from build123d import *

# Parameters (mm, degrees)
SKETCH_1_W     = 40
SKETCH_1_H     = 1.4
CHAMFER_1_SIZE = 0.2


with BuildPart() as part:
    # ｽｹｯﾁ1 → 回転1 (revolve)
    with BuildSketch(Plane(origin=(0, 0, 0), x_dir=(0, 0, -1), z_dir=(1, 0, 0)), mode=Mode.PRIVATE) as revolve_1_sk:
        with Locations((0, 2.3)):
            Rectangle(SKETCH_1_W, SKETCH_1_H)
    revolve(revolve_1_sk.sketch.rotate(Axis((0, 0, 7.128099174), (0, 0, -1)), 90), axis=Axis((0, 0, 7.128099174), (0, 0, -1)))

    # 面取り1
    chamfer_1_edges = [part.edges().sort_by_distance(p)[0] for p in [
        (-3, 0, 20),
        (-3, 0, -20),
        (-1.6, 0, -20),
        (-1.6, 0, 20),
    ]]
    chamfer(chamfer_1_edges, length=CHAMFER_1_SIZE)


solid = part.part
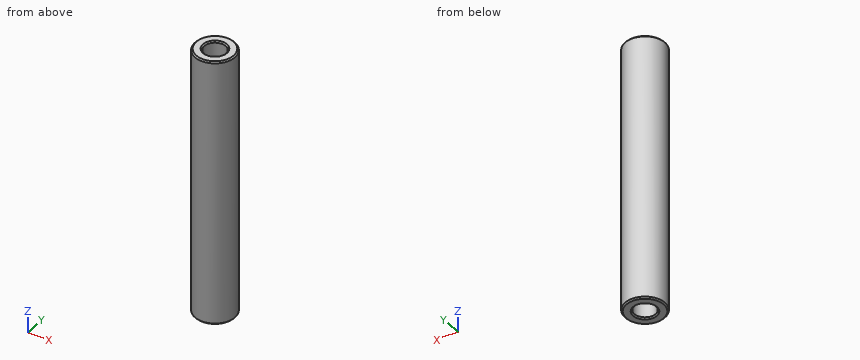
Input: part model. Units: mm. Frame: model coordinates. Coordinates: 2 decimals unless noted, no trailing zeros. Order: outer loops, then holes, each group sorted by start corner. A loop starts at its lowest first (then second) coordinate and runs counter-clockwise, first axis right, second up. Notation, with made-up numbers: M -20.75,47.5 L -0.75,47.5 A15 ccw -0.75,71.5 Z; hole C -3,76 d8. An arc over 180 degrees is marked long. Write item = value, one per line. Start each with the question number.
(1) First-contact query: P1, Ø1.5, axis at x = 0.5, y = 1.5, coming from the +Z side; P2, Ø1, axis at y = 1.5, z = 3.5, coming from the +X side. Flat tips, straight axial feed; report the tip coordinate or a pass-through.
(2) Section A-A on y = 0. Output: boundary loops of the cut face in (x, z), and give its area (3 significant figures).
(3) Section C-C on z = 15. Output: boundary loops of the cut face in (x, y), and give its area (3 significant figures).
(4) Line query: line 1 along Y through (x, z) = (0, 1.5); line 2 along X through (y, z) = (-1.25, 9); line 3 along X through (y, z) = (-0.75, 6.5). Output: solid intervals per line, ascending. Write a range as [from, to].
Result set:
q1.P1 = 20
q1.P2 = 2.83
q2.outline = M -3,-19.8 L -2.8,-20 L -1.8,-20 L -1.6,-19.8 L -1.6,19.8 L -1.8,20 L -2.8,20 L -3,19.8 Z; M 1.6,-19.8 L 1.8,-20 L 2.8,-20 L 3,-19.8 L 3,19.8 L 2.8,20 L 1.8,20 L 1.6,19.8 Z
q2.area = 112 mm²
q3.outline = C 0,0 d6; hole C 0,0 d3.2
q3.area = 20.2 mm²
q4.line_1 = [-3, -1.6], [1.6, 3]
q4.line_2 = [-2.73, -1], [1, 2.73]
q4.line_3 = [-2.9, -1.41], [1.41, 2.9]
